Here's how the part is built. I have some questions about the finished solid (model axes, mm). Give positions to 0.01 mm unless a question says otherwise; leave off trailing zeros. Loops run counter-clockwise (first coordinate to the right, second up) from the corner with the lowest first, then second, coordinate; pieces in that order, holes last. Notation, with made-up numbers: (31, 46.5) - (61, 46.5) arc R22 ccw to (61, 84.5) - close; hole circle Ø11 at (-25, 8). An arc over 180 degrees is marked (long way). Use a Markdown table: item, result.
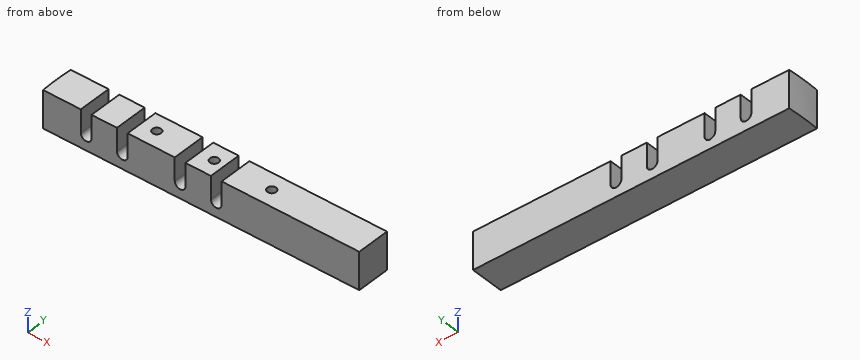
from build123d import *

# Parameters (mm, degrees)
BOSS_EXTRUDE2_DEPTH = 13.97
CUT_EXTRUDE1_DEPTH  = 9.636
SKETCH4_W           = 0.89408
SKETCH4_H           = 14.808934263
CUT_EXTRUDE2_DEPTH  = 9.636
SKETCH5_W           = 110.36886563
SKETCH5_H           = 6.670389245
CUT_EXTRUDE3_DEPTH  = 9.636
SKETCH6_R           = 1.1303
CUT_EXTRUDE4_DEPTH  = 5.08


with BuildPart() as part:
    # Sketch2 → Boss-Extrude2 (new body)
    with BuildSketch(Plane.XY):
        with BuildLine():
            Line((7.49808, 4.318), (-75.823148128, 4.318))
            ThreePointArc((-75.823148128, 4.318), (-75.946, 0), (-75.823148128, -4.318))
            Line((-75.823148128, -4.318), (7.49808, -4.318))
            Line((7.49808, -4.318), (7.49808, 4.318))
        make_face()
    extrude(amount=BOSS_EXTRUDE2_DEPTH)

    # Sketch3 → Cut-Extrude1 (cut, through all)
    with BuildSketch(Plane(origin=(0, -4.318, 0), x_dir=(-1, 0, 0), z_dir=(0, -1, 0))):
        with BuildLine():
            Line((63.17742, -10.2235), (63.17742, -3.7465))
            ThreePointArc((63.17742, -3.7465), (64.57442, -2.3495), (65.97142, -3.7465))
            Line((65.97142, -3.7465), (65.97142, -10.2235))
            ThreePointArc((65.97142, -10.2235), (64.57442, -11.6205), (63.17742, -10.2235))
        make_face()
        with BuildLine():
            Line((29.26842, -10.2235), (29.26842, -3.7465))
            ThreePointArc((29.26842, -3.7465), (30.66542, -2.3495), (32.06242, -3.7465))
            Line((32.06242, -3.7465), (32.06242, -10.2235))
            ThreePointArc((32.06242, -10.2235), (30.66542, -11.6205), (29.26842, -10.2235))
        make_face()
        with BuildLine():
            Line((38.69182, -10.2235), (38.69182, -3.7465))
            ThreePointArc((38.69182, -3.7465), (40.08882, -2.3495), (41.48582, -3.7465))
            Line((41.48582, -3.7465), (41.48582, -10.2235))
            ThreePointArc((41.48582, -10.2235), (40.08882, -11.6205), (38.69182, -10.2235))
        make_face()
        with BuildLine():
            Line((53.75402, -10.2235), (53.75402, -3.7465))
            ThreePointArc((53.75402, -3.7465), (55.15102, -2.3495), (56.54802, -3.7465))
            Line((56.54802, -3.7465), (56.54802, -10.2235))
            ThreePointArc((56.54802, -10.2235), (55.15102, -11.6205), (53.75402, -10.2235))
        make_face()
    extrude(amount=-CUT_EXTRUDE1_DEPTH, mode=Mode.SUBTRACT)

    # Sketch4 → Cut-Extrude2 (cut, through all)
    with BuildSketch(Plane.XZ.offset(4.318)):
        with Locations((7.05104, 6.565532869)):
            Rectangle(SKETCH4_W, SKETCH4_H)
    extrude(amount=-CUT_EXTRUDE2_DEPTH, mode=Mode.SUBTRACT)

    # Sketch5 → Cut-Extrude3 (cut, through all)
    with BuildSketch(Plane.XZ.offset(4.318)):
        with Locations((-32.153676927, 13.032670326)):
            Rectangle(SKETCH5_W, SKETCH5_H)
    extrude(amount=-CUT_EXTRUDE3_DEPTH, mode=Mode.SUBTRACT)

    # Sketch6 → Cut-Extrude4 (cut)
    with BuildSketch(Plane.XY.offset(9.697475704)):
        with Locations((-49.784, 0)):
            Circle(SKETCH6_R)
        with Locations((-34.798, 0)):
            Circle(SKETCH6_R)
        with Locations((-19.812, 0)):
            Circle(SKETCH6_R)
    extrude(amount=-CUT_EXTRUDE4_DEPTH, mode=Mode.SUBTRACT)


solid = part.part
(1) Will these pins go through, and if not, where does the flat tip stop? pin 1 (3 mm diameter, centred on y = -3.5, z = 7.5, fed in from -X); pin 2 (1.1 mm diameter, centred on x = -34.5, y = 0, fed in from +Z).
A:
| item | result |
|---|---|
| pin 1 | x = -75.92 |
| pin 2 | z = 4.62 |
(2) If I drill on line 1 (X direction, y = 1, z = 4); line 2 (X direction, y = 4.25, z = 9); line 3 (Y direction, x = -50, z = 7), over which ranges is the centre line in solid material (lowest first)?
A:
| item | result |
|---|---|
| line 1 | -75.94 to -65.97, -63.18 to -56.55, -53.75 to -41.49, -38.69 to -32.06, -29.27 to 6.6 |
| line 2 | -75.83 to -65.97, -63.18 to -56.55, -53.75 to -41.49, -38.69 to -32.06, -29.27 to 6.6 |
| line 3 | -4.32 to -1.11, 1.11 to 4.32 |
(3) Suppose I cut it at A-A on z = 8.75. Write out the boundary of the cut face in (x, y), plus the area to 3 significant figures.
A:
| item | result |
|---|---|
| outline | (-75.82, -4.32) - (-65.97, -4.32) - (-65.97, 4.32) - (-75.82, 4.32) arc R75.95 ccw to start; (-63.18, -4.32) - (-56.55, -4.32) - (-56.55, 4.32) - (-63.18, 4.32) - close; (-53.75, -4.32) - (-41.49, -4.32) - (-41.49, 4.32) - (-53.75, 4.32) - close; (-38.69, -4.32) - (-32.06, -4.32) - (-32.06, 4.32) - (-38.69, 4.32) - close; (-29.27, -4.32) - (6.6, -4.32) - (6.6, 4.32) - (-29.27, 4.32) - close; hole circle Ø2.26 at (-49.78, 0); hole circle Ø2.26 at (-34.8, 0); hole circle Ø2.26 at (-19.81, 0) |
| area | 604 mm2 |
